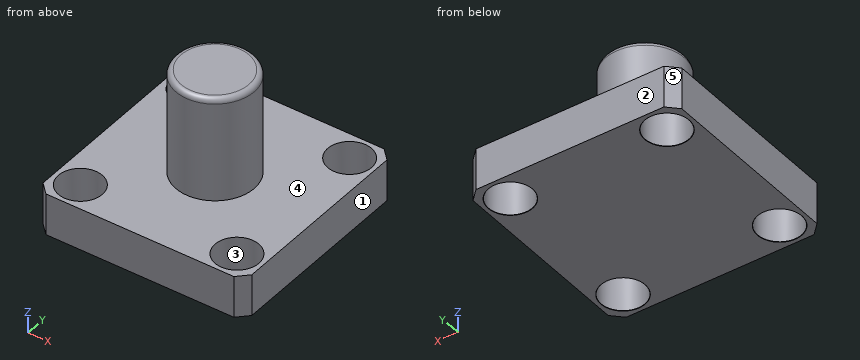
```python
from build123d import *

# Parameters (mm, degrees)
SKETCH_1_W                        = 20
SKETCH_1_H                        = 20
EXTRUDE_1_DEPTH                   = 4
SKETCH_2_R                        = 3.75
EXTRUDE_2_DEPTH                   = 10
HOLE_WIZARD_4_2_4_2_1_D           = 4.2
HOLE_WIZARD_4_2_4_2_1_CSINK_D     = 4.25
HOLE_WIZARD_4_2_4_2_1_CSINK_ANGLE = 90
FILLET_1_R                        = 0.5
CHAMFER_1_SIZE                    = 1


with BuildPart() as part:
    # 草图1 → 凸台-拉伸1 (new body)
    with BuildSketch(Plane.XY):
        Rectangle(SKETCH_1_W, SKETCH_1_H)
    extrude(amount=EXTRUDE_1_DEPTH)

    # 草图2 → 凸台-拉伸2 (add)
    with BuildSketch(Plane.XY.offset(4)):
        Circle(SKETCH_2_R)
    extrude(amount=EXTRUDE_2_DEPTH)

    # Ø4.2 (4.2) 直径孔1 (through all)
    with Locations(Plane(origin=(7.5, 7.5, 0), x_dir=(-1, 0, 0), z_dir=(0, 0, -1))):
        with Locations((0, 0), (15, 0), (15, -15), (0, -15)):
            CounterSinkHole(HOLE_WIZARD_4_2_4_2_1_D / 2, HOLE_WIZARD_4_2_4_2_1_CSINK_D / 2, counter_sink_angle=HOLE_WIZARD_4_2_4_2_1_CSINK_ANGLE)

    # 圆角1
    fillet_1_edges = [part.edges().sort_by_distance(p)[0] for p in [
        (-3.75, 0, 14),
    ]]
    fillet(fillet_1_edges, radius=FILLET_1_R)

    # 倒角1
    chamfer_1_edges = [part.edges().sort_by_distance(p)[0] for p in [
        (10, -10, 2),
        (-10, -10, 2),
        (-10, 10, 2),
        (10, 10, 2),
    ]]
    chamfer(chamfer_1_edges, length=CHAMFER_1_SIZE)


solid = part.part
```
Input: part model. Units: mm. Frame: model coordinates. Face numbers are marked on the shaded views. A direction names the side the tool comes from. Round coordinates to 2 decimals unless told otherwise and drop trailing zeros. Order: outer loops, then holes, each group sorted by start corner. A loop starts at its lowest first (then second) coordinate and runs counter-clockwise, first axis right, second up. Notation, with made-up numbers: (74.25, 68) - (104.25, 68) arc R10 cw to (104.25, 86) - close; hole circle Ø5 at (-11.5, 44). An arc over 180 degrees is marked (long way). One line per question, with ' | ' between items. Start each with the question number.
1) Set-up query: the marked faces 4 and 5. Return all of +Z, -Z, +X, -X, +Y, -Y with unobstructed straight access to the full face (end or side cutting, diameter ignored); none if empty.
2) Contact query for flat-ended pins moving along their axis: P1, Ø4, axis at y = 1, z = 8.5, coming from the +X side; P2, Ø4, axis at y = 6, z = 12.5, coming from the +X side; P3, Ø6.5, axis at x = 7.5, y = 7.5, coming from the +Z side. Output: stop coordinate, or through.
3) Ray query, probe 1 along X at (y, z) = (-7.5, 2.45); probe 2 along Z at (x, y) = (0.5, -4). Return the intervals inside material, ascending.
4) Cut plane A-A, the plane x = 7.5. Return the cut outline in (y, z) (3 decimals), then the cut area to 3 significant figures.
5) Cut plane C-C, the plane z = 1.5. Return the cut outline in (x, y).
6) Pull-direction query (Y, two-part tool) for the marked faces 1, 2 and 3; classes: +Y half, -Y half, draft (parallel to the pull), parting line (faces both ways), or undercut.
7) Cut plane D-D, the plane x = 0. Return the cut outline in (y, z), then the cut area to 3 significant figures.
Worked out:
1) face 4: +Z | face 5: +Z, -Z, -X, +Y
2) P1: stops at x = 3.75 | P2: passes through | P3: stops at z = 4
3) probe 1: x = -10 to -9.6, -5.4 to 5.4, 9.6 to 10 | probe 2: z = 0 to 4
4) outline: (-10, 0) - (-9.625, 0) - (-9.6, 0.025) - (-9.6, 4) - (-10, 4) - close; (-5.4, 0.025) - (-5.375, 0) - (5.375, 0) - (5.4, 0.025) - (5.4, 4) - (-5.4, 4) - close; (9.6, 0.025) - (9.625, 0) - (10, 0) - (10, 4) - (9.6, 4) - close | area: 46.4 mm^2
5) outline: (-10, -9) - (-9, -10) - (9, -10) - (10, -9) - (10, 9) - (9, 10) - (-9, 10) - (-10, 9) - close; hole circle Ø4.2 at (-7.5, -7.5); hole circle Ø4.2 at (-7.5, 7.5); hole circle Ø4.2 at (7.5, -7.5); hole circle Ø4.2 at (7.5, 7.5)
6) face 1: draft | face 2: +Y half | face 3: undercut
7) outline: (-10, 0) - (10, 0) - (10, 4) - (3.75, 4) - (3.75, 13.5) arc R0.5 ccw to (3.25, 14) - (-3.25, 14) arc R0.5 ccw to (-3.75, 13.5) - (-3.75, 4) - (-10, 4) - close | area: 155 mm^2
